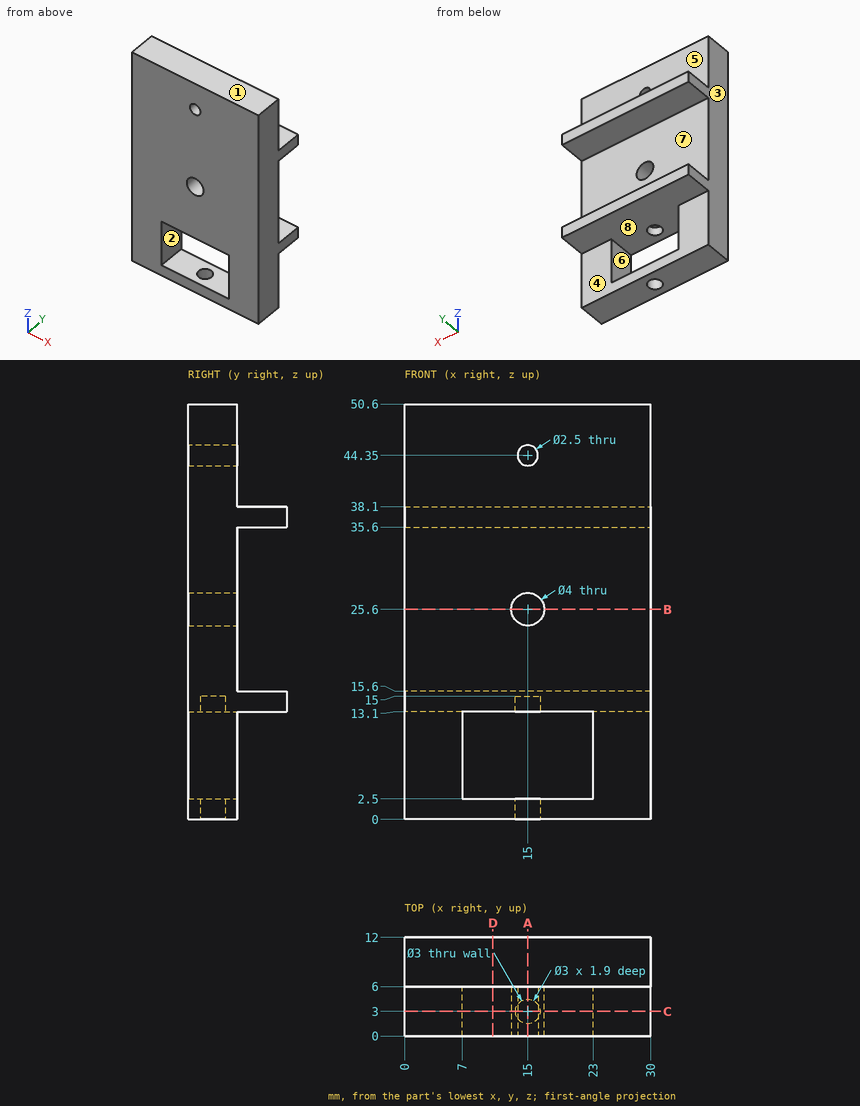
Answer from the drawing. Dimensions are ordinates in mm from the lowest x, y and z of the part. A direction names the side the tool comes from. Coordinates: 2 decimals unless noted, no trailing zeros. Loops run counter-clockwise (first coordinate to the right, second up) from the corner with the lowest first, then second, coordinate; pieces in that order, holes last.
Q1. This flat-tipped pin is pushed along its axis until it touches: pin 1 Ø4.5 at (x, z) = (15, 25.6) entering from +Y. Where does it stop, or does it pass through?
Q2. The part is cut by section C-C on y = 3. Write down the section's boundary in (x, z).
Q3. The part is cut by section A-A on x = 15. Give the number of separate pieces and of enclosed holes in the cut face, and give its area (3 significant figures).
Q4. Consider probe 1 along Z at (x, y) = (15, 2.1); probe 2 along Z at (x, y) = (16, 9.25); probe 3 along Y at (x, z) = (15, 1.9). Determine where each line is inside the solid, lowest interval first.
Q5. The part is cut by section D-D on x = 10.75. Write down the section's boundary in (y, z), and give its area (3 significant figures).
Q6. Which of the six approach directions +Z, -Z, +X, -X, +Y, -Y give full straight-line access (tool end or side, diameter ignored) to the marked faces 4, 5, 6, 7 and 8?
Q7. The mould has two halves that part along X. Classify the marked faces 1, 2 and 3: +X half, -X half, draft (parallel to the pull), parting line (faces both ways), or undercut.
Q8. The part is cut by section B-B on z = 25.6. Write down the section's boundary in (x, y), and give its area (3 significant figures).
Results below:
1. pin 1: stops at y = 6
2. outline: (0, 0) - (13.5, 0) - (13.5, 2.5) - (7, 2.5) - (7, 13.1) - (13.5, 13.1) - (13.5, 15) - (16.5, 15) - (16.5, 13.1) - (23, 13.1) - (23, 2.5) - (16.5, 2.5) - (16.5, 0) - (30, 0) - (30, 50.6) - (0, 50.6) - close; hole circle Ø4 at (15, 25.6); hole circle Ø2.5 at (15, 44.35)
3. separate pieces: 5
3. enclosed holes: 0
3. area: 218 mm2
4. probe 1: z = 15 to 23.6, 27.6 to 43.1, 45.6 to 50.6
4. probe 2: z = 13.1 to 15.6, 35.6 to 38.1
4. probe 3: y = 0 to 1.5, 4.5 to 6
5. outline: (0, 0) - (6, 0) - (6, 2.5) - (0, 2.5) - close; (0, 13.1) - (12, 13.1) - (12, 15.6) - (6, 15.6) - (6, 35.6) - (12, 35.6) - (12, 38.1) - (6, 38.1) - (6, 50.6) - (0, 50.6) - close
5. area: 270 mm2
6. face 4: -Z, +X, -X, +Y
6. face 5: +Z, +X, -X, +Y
6. face 6: +Y, -Y
6. face 7: +X, -X, +Y
6. face 8: +Y
7. face 1: draft
7. face 2: undercut
7. face 3: -X half
8. outline: (0, 0) - (13, 0) - (13, 6) - (0, 6) - close; (17, 0) - (30, 0) - (30, 6) - (17, 6) - close
8. area: 156 mm2
